Autodesk Inventor part; units mm, degrees
ref_plane "YZ Plane" through (0, 0, 0) normal (1, 0, 0) x (0, 1, 0)
ref_plane "XZ Plane" through (0, 0, 0) normal (0, 1, 0) x (-1, 0, 0)
ref_plane "XY Plane" through (0, 0, 0) normal (0, 0, 1) x (1, 0, 0)
sketch "Sketch1" plane through (0, 0, 0) normal (0, 0, 1) x (1, 0, 0)
  line L0 (0, 0) -> (38.1, 0)
  line L1 (38.1, 0) -> (38.1, 253.0348)
  arc A0 (38.1, 507.0348) -> (38.1, 253.0348) centre (666.75, 380.0348) ccw
  line L2 (38.1, 507.0348) -> (38.1, 608.6348)
  line L3 (38.1, 608.6348) -> (0, 608.6348)
  line L4 (0, 608.6348) -> (0, 0)
  circle A1 centre (31.75, 151.4348) radius 3.3655
  circle A2 centre (31.75, 34.671) radius 3.3655
  circle A3 centre (12.7, 12.7) radius 3.3655
  circle A4 centre (12.7, 342.9) radius 3.3655
  circle A5 centre (12.7, 595.9348) radius 3.3655
  circle A6 centre (31.75, 12.7) radius 3.3655
  circle A7 centre (31.75, 253.0348) radius 3.3655
  circle A8 centre (31.75, 507.0348) radius 3.3655
  circle A9 centre (31.75, 595.9348) radius 3.3655
  line L5 (0, 557.8348) -> (0, 608.6348)
  line L6 (0, 50.8) -> (0, 0)
  line L7 (12.7, 342.9) -> (0, 304.3174) construction
  line L8 (0, 317.5) -> (0, 368.3)
  line L9 (0, 129.921) -> (12.7, 129.921) construction
  circle A10 centre (12.7, 129.921) radius 3.3655
  circle A11 centre (12.7, 174.371) radius 3.3655
  line L10 (9.3413, 197.482) -> (9.3413, 204.213)
  line L11 (16.0611, 204.488) -> (16.0611, 197.3435)
  arc A12 (16.0611, 204.488) -> (9.3413, 204.213) centre (12.6956, 204.488) ccw
  arc A13 (9.3413, 197.482) -> (16.0611, 197.3435) centre (12.6974, 197.231) ccw
  circle A14 centre (12.7, 217.188) radius 3.3655
  dimension "d0" = 38.1
  dimension "d2" = 101.6
  dimension "d4" = 457.2
  dimension "d5" = 101.6
  dimension "d6" = 666.75
  dimension "d7" = 641.35
  dimension "d9" = 116.7638
  dimension "d10" = 6.35
  dimension "d11" = 6.35
  dimension "d13" = 12.7
  dimension "d14" = 12.7
  dimension "d16" = 12.7
  dimension "d17" = 342.9
  dimension "d19" = 12.7
  dimension "d20" = 12.7
  dimension "d22" = 6.35
  dimension "d24" = 6.35
  dimension "d25" = 6.731
  dimension "d26" = 6.35
  dimension "hole" = 6.731
  dimension "d28" = 6.35
  dimension "d45" = 12.7
  dimension "d47" = 12.7
  dimension "d54" = 6.731
  dimension "d55" = 3.3655
  dimension "d56" = 3.3655
  dimension "d58" = 6.731
  dimension "d59" = 12.7
  dimension "d68" = 18.22
  dimension "d69" = 90
  dimension "d70" = 90
  dimension "d71" = 22.0389
  dimension "d72" = 28.7587
  dimension "d73" = 478.7138
  dimension "d74" = 6.35
  dimension "d75" = 6.35
  dimension "d76" = 595.9348
  dimension "d77" = 404.1468
  dimension "d78" = 411.2913
  dimension "d79" = 25.4
  dimension "d80" = 25.4
  dimension "d81" = 434.2638
  dimension "d82" = 50.8
  dimension "d83" = 240.3348
  dimension "d84" = 291.1348
  dimension "d85" = 557.8348
extrude "Plate4" add sketch "Sketch1" along normal blind 3.048
sketch "Sketch5" plane through (0, 0, 3.048) normal (0, 0, 1) x (1, 0, 0)
  line L0 (38.1, 0) -> (38.1, 253.0348)
  line L1 (0, 0) -> (38.1, 0)
  line L2 (38.1, 0) -> (38.1, 25.4)
  line L3 (38.1, 25.4) -> (0, 25.4)
  line L4 (0, 25.4) -> (0, 0)
  dimension "d96" = 25.4
extrude "Cut1" cut sketch "Sketch5" against normal blind 3.048
sketch "Sketch7" plane through (0, 25.4, 3.048) normal (-1, 0, 0) x (0, -1, 0)
  line L0 (-583.2348, 0) -> (0, 0)
  line L1 (0, 0) -> (0, 22.352)
  line L2 (0, 22.352) -> (-583.2348, 22.352)
  line L3 (-583.2348, 22.352) -> (-583.2348, 0)
edge flange "Flange3" height 25.4 angle 90 thickness 3.048 bend radius 3.048 thickness toward (-1, 0, 0) relief tear relief width 3.048 relief depth 1.524 edges at (0, 317.0174, 3.048) wall of the first edge with corners at (0, 608.6348, 3.048) (0, 25.4, 3.048) (0, 25.4, 25.4) (0, 608.6348, 25.4)
bend "Bend3"
corner "Corner3"
sketch "Sketch8" plane through (-3.048, 25.4, 25.4) normal (0, -1, 0) x (1, 0, 0)
  line L0 (0, 0) -> (41.148, 0)
  line L1 (41.148, 0) -> (41.148, -25.4)
  line L2 (41.148, -25.4) -> (0, -25.4)
  line L3 (0, -25.4) -> (0, 0)
  point P0 (3.048, -25.4)
extrude "Extrusion1" cut sketch "Sketch8" against normal blind 222.25
equation "\"d25\" = hole"
equation "\"d97\" = Thickness"
equation "\"d109\" = BendReliefWidth"
equation "\"d110\" = BendReliefDepth"
equation "\"d111\" = MinimumRemnant"
equation "\"d112\" = BendRadius"
equation "\"d115\" = BendRadius"
equation "\"d116\" = CornerReliefSize"
equation "\"d117\" = GapSize"
equation "\"d118\" = JacobiRadiusSize"
equation "\"BendRadius\" = Thickness"
equation "\"BendReliefWidth\" = Thickness"
equation "\"BendReliefDepth\" = 0.5 * Thickness"
equation "\"CornerReliefSize\" = 4 * Thickness"
equation "\"MinimumRemnant\" = 2 * Thickness"
equation "\"TransitionRadius\" = BendRadius"
equation "\"JacobiRadiusSize\" = BendRadius"
equation "\"GapSize\" = Thickness"
equation "\"d29\" = BendRadius"
equation "\"d32\" = BendRadius"
equation "\"d38\" = BendRadius"
equation "\"d60\" = BendRadius"
properties part number "Claw - Arm - Top (R) Bottom"
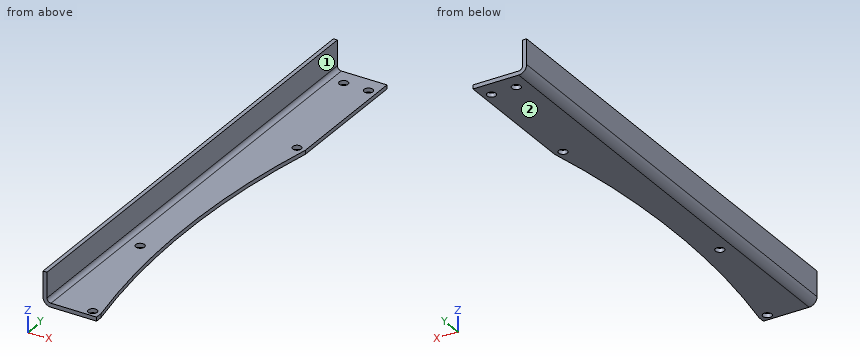
Could you check a few things on this model? Use its own coordinates, in mm. Face numbers are marked on the shaded views. A direction names the side the tool comes from. Give positions to 0.01 mm unless a question says otherwise; leave off trailing zeros. Write each loop counter-clockwise with the first axis right and the second up, starting at its lowest first coordinate (ties: lowest second). Pieces come first, ordered by that corner, then holes. Notation, with made-up numbers: (69.25, 38) -> (74.25, 38) arc R23 ccw to (74.25, 60) -> close; hole circle Ø9 at (-20.75, 73.25). An arc over 180 degrees is marked (long way). Answer as CSV lines item,"result". Start each with the question number.
(1) If we section it at B-B, the plane y = 542.5: Write out the boundary of the cut face in (x, z).
(2) Which directions (+Z, -Z, +X, -X, +Y, -Y) give clear straight access to the entire face, cutting with the end or side of a thin tool? Please do the marked faces 1 and 2.
(3) If we section it at A-A, the plane x = 12.7: Write out the boundary of the cut face in (y, z).
(4) If we section it at D-D, the plane y = 342.9: Write out the boundary of the cut face in (x, z), and give its area (3 significant figures).
(5) If we section it at C-C, the plane x = 31.75: Write out the boundary of the cut face in (y, z), and give its area (3 significant figures).
(6) I'm going to push flat-ended pins straight in: pin 1 Ø6 at (x, y) = (17, 401) entering from +Z; pin 2 Ø5.5 at (x, y) = (31.75, 507.03) entering from +Z; pin 3 Ø9.5 at (y, z) = (516, 14) entering from +X. Where does each tip first touch, or does it pass through?
(7) Please list where these lines run through material, in increasing order: line 1 (Y direction, x = 12.7, z = 1.3); line 2 (Y direction, x = 11, z = 1.75); line 3 (X direction, y = 305, z = 23.5).
Answer list:
1,outline,"(-3.05, 6.1) arc R6.1 ccw to (3.05, 0) -> (38.1, 0) -> (38.1, 3.05) -> (3.05, 3.05) arc R3.05 cw to (0, 6.1) -> (0, 25.4) -> (-3.05, 25.4) -> close"
2,face 1,"+Z, +X, +Y, -Y"
2,face 2,"-Z, +X, -X, +Y, -Y"
3,outline,"(247.65, 0) -> (339.53, 0) -> (339.53, 3.05) -> (247.65, 3.05) -> close; (346.27, 0) -> (592.57, 0) -> (592.57, 3.05) -> (346.27, 3.05) -> close; (599.3, 0) -> (608.63, 0) -> (608.63, 3.05) -> (599.3, 3.05) -> close"
4,outline,"(-3.05, 6.1) arc R6.1 ccw to (3.05, 0) -> (9.33, 0) -> (9.33, 3.05) -> (3.05, 3.05) arc R3.05 cw to (0, 6.1) -> (0, 25.4) -> (-3.05, 25.4) -> close; (16.07, 0) -> (26.48, 0) -> (26.48, 3.05) -> (16.07, 3.05) -> close"
4,area,"132 mm^2"
5,outline,"(247.65, 0) -> (249.67, 0) -> (249.67, 3.05) -> (247.65, 3.05) -> close; (256.4, 0) -> (290.01, 0) -> (290.01, 3.05) -> (256.4, 3.05) -> close; (470.06, 0) -> (503.67, 0) -> (503.67, 3.05) -> (470.06, 3.05) -> close; (510.4, 0) -> (592.57, 0) -> (592.57, 3.05) -> (510.4, 3.05) -> close; (599.3, 0) -> (608.63, 0) -> (608.63, 3.05) -> (599.3, 3.05) -> close"
5,area,"490 mm^2"
6,pin 1,"z = 3.05"
6,pin 2,"through"
6,pin 3,"x = 0"
7,line 1,"247.65 to 339.53, 346.27 to 592.57, 599.3 to 608.63"
7,line 2,"247.65 to 340, 345.8 to 593.03, 598.84 to 608.63"
7,line 3,"-3.05 to 0"
